```python
from build123d import *

# Parameters (mm, degrees)
F0_W       = 24
F0_H       = 24
F1_DEPTH   = 60
F4_D       = 8
F4_ON_F2_D = 8


with BuildPart() as f1:
    # F0 (on Front) → F1 (new body)
    with BuildSketch(Plane.XZ):
        Rectangle(F0_W, F0_H)
    extrude(amount=F1_DEPTH)

    # F4 (through all)
    with Locations(Plane.YZ.offset(12)):
        with Locations((-12, 0)):
            Hole(F4_D / 2)

    # F4 on F2 (through all)
    with Locations(Plane(origin=(0, 0, -12), x_dir=(1, 0, 0), z_dir=(0, 0, -1))):
        with Locations((0, 48)):
            Hole(F4_ON_F2_D / 2)


solid = f1.part
```
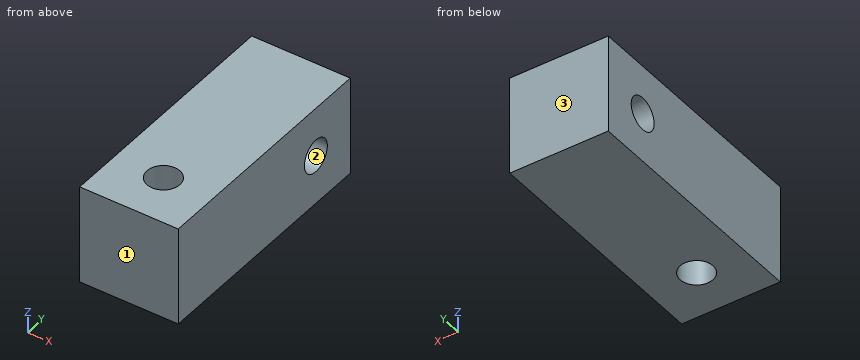
The listing builds one solid part. Answer for the finished solid, in the listing's coordinates (mm). Face numbers are marked on the shaded views. Coordinates: 2 decimals unless noted, no trailing zeros. Write each loop counter-clockwise with the first axis right and the second up, starting at its lowest first coordinate (ties: lowest second). Pieces come first, ordered by that corner, then holes.
Q1. The mould has two halves that part along Y. Classify the marked faces 1, 2 and 3: released by +Y, released by -Y, zero draft, split by the parting line, or undercut.
Returned:
face 1: released by -Y
face 2: undercut
face 3: released by +Y
Q2. Section D-D, the plane z = -8.75 is taken. Write down the section's boundary in (x, y), then the cut area to 3 significant figures.
Returned:
outline: (-12, -60) - (12, -60) - (12, 0) - (-12, 0) - close; hole circle Ø8 at (0, -48)
area: 1,390 mm2
Q3. Section B-B, the plane x = 0 is taken. Write down the section's boundary in (y, z).
Returned:
outline: (-60, -12) - (-52, -12) - (-52, 12) - (-60, 12) - close; (-44, -12) - (0, -12) - (0, 12) - (-44, 12) - close; hole circle Ø8 at (-12, 0)
Q4. Find the intervals of material crossed by line 1 along Z through (x, y) = (1.5, -12); line 2 along X through (y, z) = (-51, 5.75), in increasing order.
Returned:
line 1: z = -12 to -4, 4 to 12
line 2: x = -12 to -2.65, 2.65 to 12
Q5. Section C-C, the plane y = -12 is taken. Write down the section's boundary in (x, z).
Returned:
outline: (-12, -12) - (12, -12) - (12, -4) - (-12, -4) - close; (-12, 4) - (12, 4) - (12, 12) - (-12, 12) - close
Q6. Section A-A, the plane z = 0 is taken. Write down the section's boundary in (x, y).
Returned:
outline: (-12, -60) - (12, -60) - (12, -16) - (-12, -16) - close; (-12, -8) - (12, -8) - (12, 0) - (-12, 0) - close; hole circle Ø8 at (0, -48)
